Source: CAD feature listing. Evaluate the final solid. Frame: model axes, mm. A direction names the side the tool comes from. Give positions to 0.01 mm unless a question says otherwise; leave off trailing zeros. Loops run counter-clockwise (first coordinate to the right, second up) from the corner with the lowest first, then second, coordinate; pieces in that order, holes last. Notation, with made-up numbers: M 38,-18.5 L 67,-18.5 A31 cw 67,18.5 Z; hole C 53,16 d10. An arc over 180 degrees is marked long. Put each result on its own line as item: value.
from build123d import *

# Parameters (mm, degrees)
SKETCH_1_W               = 4
SKETCH_1_H               = 27.5
CUT_EXTRUDE_4_DEPTH      = 71.823724839
CUT_EXTRUDE_4_DEPTH_BACK = 71.823724839
SKETCH_7_R               = 50
SKETCH_7_W               = 60
SKETCH_7_H               = 60
CUT_EXTRUDE_3_DEPTH      = 43.614551505
PATTERN_CIRCULAR_2_COUNT = 4
FILLET_1_R               = 3


with BuildPart() as part:
    # Эскиз1 → Повернуть1 (revolve)
    with BuildSketch(Plane.XY, mode=Mode.PRIVATE) as revolve_1_sk:
        with Locations((2, 36.25)):
            Rectangle(SKETCH_1_W, SKETCH_1_H)
    revolve(revolve_1_sk.sketch.rotate(Axis((-29.36512031, 0, 0), (1, 0, 0)), 90), axis=Axis((-29.36512031, 0, 0), (1, 0, 0)))

    # Эскиз7 → Вырез-Вытянуть4 (cut, two sides: drawn at the far end of the back side and taken through both)
    with BuildSketch(Plane.ZY.offset(-CUT_EXTRUDE_4_DEPTH_BACK)):
        Circle(SKETCH_7_R)
        Rectangle(SKETCH_7_W, SKETCH_7_H, mode=Mode.SUBTRACT)
    extrude(amount=CUT_EXTRUDE_4_DEPTH + CUT_EXTRUDE_4_DEPTH_BACK, mode=Mode.SUBTRACT)

    # Эскиз6 → Вырез-Вытянуть3 (cut, symmetric)
    with BuildSketch(Plane.ZY):
        with BuildLine():
            Line((-27.192031022, 24.222182541), (-25.777817459, 22.807968978))
            ThreePointArc((-25.777817459, 22.807968978), (-22.807968978, 22.807968978), (-22.807968978, 25.777817459))
            Line((-22.807968978, 25.777817459), (-24.222182541, 27.192031022))
            ThreePointArc((-24.222182541, 27.192031022), (-27.192031022, 27.192031022), (-27.192031022, 24.222182541))
        make_face()
    cut_extrude_3 = extrude(amount=CUT_EXTRUDE_3_DEPTH, both=True, mode=Mode.SUBTRACT)

    # Круговой массив2: Вырез-Вытянуть3 ×4 about axis
    pattern_circular_2_axis = Axis((0, 0, 0), (1, 0, 0))
    for i in range(1, PATTERN_CIRCULAR_2_COUNT):
        add(cut_extrude_3.rotate(pattern_circular_2_axis, i * 360 / PATTERN_CIRCULAR_2_COUNT), mode=Mode.SUBTRACT)

    # Скругление1
    fillet_1_edges = [part.edges().sort_by_distance(p)[0] for p in [
        (2, 30, -30),
        (2, 30, 30),
        (2, -30, 30),
        (2, -30, -30),
    ]]
    fillet(fillet_1_edges, radius=FILLET_1_R)


solid = part.part
1. Section query A-A (z = 0). Output: boundary loops of the cut face in (x, y), plus the area to 3 significant figures.
Found:
outline: M 0,-30 L 4,-30 L 4,-22.5 L 0,-22.5 Z; M 0,22.5 L 4,22.5 L 4,30 L 0,30 Z
area: 60.0 mm^2
2. Material intervals for line 1 (Y direction, x = 2.95, z = 0); line 2 (Z direction, x = 3.65, y = 23.5); line 3 (Y direction, x = 2.3, z = -15), sorted ascending. Write a range as from..to.
Found:
line 1: -30..-22.5, 22.5..30
line 2: -30..-26.47, -22.35..22.35, 26.47..30
line 3: -30..-16.77, 16.77..30
3. Access query for faces 1 (the flat face through (1.97, 23.51, 26.48)), 2 (the cylindrical face through (1.97, -29.14, -29.1)). Directions: +Z, -Z, +X, -X, +Y, -Y. A direction counts if a zero-diameter tool reaches every point of the face in a straight line with its end or side. Return the directions, or none.
Found:
face 1: +X, -X
face 2: -Z, +X, -X, -Y
4. Draft query along Z for faces 3 (the cylindrical face through (1.97, -29.14, 29.1)), 4 (the flat face through (1.97, -23.52, 26.49)), 5 (the flat face through (2, 0, -30)). Return one class per face: pulls with the +Z half, pulls with the -Z half, needs draft (parallel to the pull), parting line crosses it, or undercut.
Found:
face 3: pulls with the +Z half
face 4: undercut
face 5: pulls with the -Z half
5. Section query C-C (x = 0.7). Output: boundary loops of the cut face in (y, z).
Found:
outline: M -30,-27 A3 ccw -27,-30 L 27,-30 A3 ccw 30,-27 L 30,27 A3 ccw 27,30 L -27,30 A3 ccw -30,27 Z; hole M -27.19,-24.22 A2.1 ccw -24.22,-27.19 L -22.81,-25.78 A2.1 ccw -25.78,-22.81 Z; hole M -27.19,24.22 L -25.78,22.81 A2.1 ccw -22.81,25.78 L -24.22,27.19 A2.1 ccw Z; hole C 0,0 d45; hole M 22.81,-25.78 L 24.22,-27.19 A2.1 ccw 27.19,-24.22 L 25.78,-22.81 A2.1 ccw Z; hole M 22.81,25.78 A2.1 ccw 25.78,22.81 L 27.19,24.22 A2.1 ccw 24.22,27.19 Z
